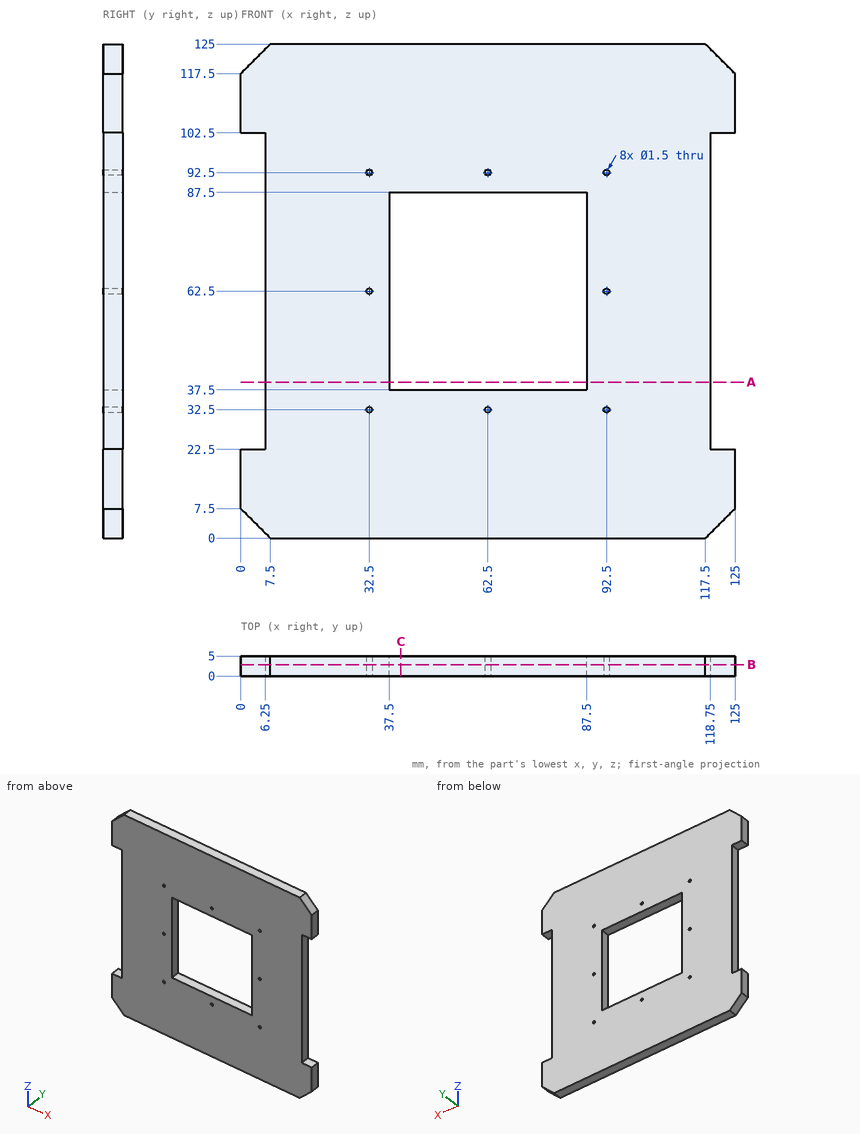
For this review, use the dimensioned drawing (mm, ordinates from the lowest corner) and the shaded views. Give positions to 0.01 mm unless a question says otherwise; leave off trailing zeros. Order: outer loops, then holes, each group sorted by start corner. A loop starts at its lowest first (then second) coordinate and runs counter-clockwise, first axis right, second up. Notation, with made-up numbers: (70.25, 20.5) - (86.25, 20.5) arc R9 ccw to (86.25, 35.5) - close; hole circle Ø8 at (-0.75, -21.5). An arc over 180 degrees is marked (long way). Use CSV: the item, a comma, the result in double quotes. Start each with the question number.
Q1. For line 1 (X direction, y = 1.9, z = 92.5); line 2 (Z direction, x = 62.5, y = 1.1); line 3 (X direction, y = 1.5, z = 62.5), list the stretches that pass through material, from the lowest coordinate up.
Q2. Take a section at A-A (z = 39.5). State the section outline as (x, y) points.
Q3. For P1, Ø2, axis at y = 3.5, z = 86, coming from the -X side; P2, Ø1.5, axis at y = 3.5, z = 86, coming from the +X side, all flat-tipped, find the tip position at first contact; note any pin that passes through.
Q4. Take a section at B-B (y = 2.85). Count the separate pieces of the cut face and the enclosed holes in it, and give its area (3 significant figures).
Q5. Take a section at C-C (x = 40.5). State the section outline as (y, z) points, and give its area (3 significant figures).
Calculated:
1,line 1,"x = 6.25 to 31.75, 33.25 to 61.75, 63.25 to 91.75, 93.25 to 118.75"
1,line 2,"z = 0 to 31.75, 33.25 to 37.5, 87.5 to 91.75, 93.25 to 125"
1,line 3,"x = 6.25 to 31.75, 33.25 to 37.5, 87.5 to 91.75, 93.25 to 118.75"
2,outline,"(6.25, 0) - (37.5, 0) - (37.5, 5) - (6.25, 5) - close; (87.5, 0) - (118.75, 0) - (118.75, 5) - (87.5, 5) - close"
3,P1,"stops at x = 6.25"
3,P2,"stops at x = 118.75"
4,separate pieces,"1"
4,enclosed holes,"9"
4,area,"12,000 mm²"
5,outline,"(0, 0) - (5, 0) - (5, 37.5) - (0, 37.5) - close; (0, 87.5) - (5, 87.5) - (5, 125) - (0, 125) - close"
5,area,"375 mm²"
